Verification items for the finished model (mm, model axes). A direction names the side the tool comes from. Give positions to 0.01 mm unless a question says otherwise; leave off trailing zeros. Loops run counter-clockwise (first coordinate to the right, second up) from the corner with the lowest first, then second, coordinate; pieces in that order, holes last. Notation, with made-up numbers: (55.5, 28) - (81.5, 28) arc R10 cw to (81.5, 37) - close; hole circle Ø2 at (25, 22). An arc over 180 degrees is marked (long way). One line per item, written item: value. Start each with the question number.
1. Sectioned sample at A-A (x = 0.5). Record the cut outline in (y, z), plus the area to 3 significant figures.
2. Gauge pin test, flat ends, axial feed: pin 1 (2 mm diameter, centred on x = 17.5, y = 17.5, fed in from -Z); pin 2 (8.5 mm diameter, centred on x = -3, y = -1.5, fed in from -Z); pin 3 (1.4 mm diameter, centred on x = 17, y = 18, fed in from -Z); pin 4 (2.5 mm diameter, centred on y = -19, z = -3, fed in from -X). Record the tip position at first contact, or that the pin passes through.
3. Sectioned sample at C-C (y = -4). Record the cut outline in (x, z), plus the area to 3 significant figures.
4. Mould release check, pull along Y, two halves, no side actions. Record for faces 1 (the flat face through (15, 14, 0)), 2 (the cylindrical face through (16.002, 15.963, 4.493)), 3 (the flat face through (15, 0, -3.85)), 4 (the flat face through (-20, 0, 0)): pulls with the +Y half, pulls with the -Y half, needs draft (parallel to the pull), parting line crosses it, or undercut.
5. Scan lines: L1, parallel to Y at x = -17.5, z = 2.9; L2, parallel to Y at x = 17.5, z = 2.95; L3, parallel to Y at x = 0.5, z = -4.4. Record each from-to range of solid material in increasing order. Write a range as [from, to].
6. Sectioned sample at B-B (z = -2.5). Record the cut outline in (x, y), plus the area to 3 significant figures.
7. Sectioned sample at D-D (y = -8.5). Record the cut outline in (x, z).
8. Access from +Z, -Z, +X, -X, +Y, -Y to the whole of each face (thin tool, end or side, straight path). Record for faces 5 (the cylindrical face through (15.963, -16.002, 4.493)), 6 (the cylindrical face through (-15.963, 16.002, -1.796)), 7 (the flat face through (-18, 19, 4)), 8 (the flat face through (-19, -18, 4)).
from build123d import *

# Parameters (mm, degrees)
SKETCH_1_W          = 40
SKETCH_1_H          = 40
EXTRUDE_1_DEPTH     = 5
SKETCH_2_W          = 7.7
SKETCH_2_H          = 28
CUT_EXTRUDE_1_DEPTH = 10
CUT_EXTRUDE_2_DEPTH = 6.5
FILLET_1_R          = 2
CUT_EXTRUDE_START   = -1
CUT_EXTRUDE_3_DEPTH = 1
CUT_EXTRUDE_4_REACH = 31.682
SKETCH_5_R          = 1.189
SKETCH_6_R          = 14
CUT_EXTRUDE_5_DEPTH = 1


with BuildPart() as part:
    # 草图1 → 凸台-拉伸1 (new, symmetric)
    with BuildSketch(Plane.XY):
        Rectangle(SKETCH_1_W, SKETCH_1_H)
    extrude(amount=EXTRUDE_1_DEPTH, both=True)

    # 草图2 → 切除-拉伸1 (cut)
    with BuildSketch(Plane(origin=(20, 0, 0), x_dir=(0, 0, -1), z_dir=(1, 0, 0))):
        Rectangle(SKETCH_2_W, SKETCH_2_H)
    extrude(amount=-CUT_EXTRUDE_1_DEPTH, mode=Mode.SUBTRACT)

    # 草图3 → 切除-拉伸2 (cut)
    with BuildSketch(Plane(origin=(0, 0, -5), x_dir=(-1, 0, 0), z_dir=(0, 0, -1))):
        with BuildLine():
            Line((20, 20), (15.25, 20))
            Line((15.25, 20), (15.25, 17.75))
            ThreePointArc((15.25, 17.75), (15.982233047, 15.982233047), (17.75, 15.25))
            Line((17.75, 15.25), (20, 15.25))
            Line((20, 15.25), (20, 20))
        make_face()
        with BuildLine():
            Line((20, -20), (20, -15.25))
            Line((20, -15.25), (17.75, -15.25))
            ThreePointArc((17.75, -15.25), (15.982233047, -15.982233047), (15.25, -17.75))
            Line((15.25, -17.75), (15.25, -20))
            Line((15.25, -20), (20, -20))
        make_face()
        with BuildLine():
            Line((-17.75, -15.25), (-20, -15.25))
            Line((-20, -15.25), (-20, -20))
            Line((-20, -20), (-15.25, -20))
            Line((-15.25, -20), (-15.25, -17.75))
            ThreePointArc((-15.25, -17.75), (-15.982233047, -15.982233047), (-17.75, -15.25))
        make_face()
        with BuildLine():
            Line((-15.25, 17.75), (-15.25, 20))
            Line((-15.25, 20), (-20, 20))
            Line((-20, 20), (-20, 15.25))
            Line((-20, 15.25), (-17.75, 15.25))
            ThreePointArc((-17.75, 15.25), (-15.982233047, 15.982233047), (-15.25, 17.75))
        make_face()
    extrude(amount=-CUT_EXTRUDE_2_DEPTH, mode=Mode.SUBTRACT)

    # 圆角1
    fillet_1_edges = [part.edges().sort_by_distance(p)[0] for p in [
        (20, -20, 3.25),
        (-20, -20, 3.25),
        (-20, 20, 3.25),
        (20, 20, 3.25),
    ]]
    fillet(fillet_1_edges, radius=FILLET_1_R)

    # 草图4 → 切除-拉伸3 (cut)
    with BuildSketch(Plane.XY.offset(5).offset(CUT_EXTRUDE_START)):
        with BuildLine():
            Line((20, -15.25), (20, -18))
            ThreePointArc((20, -18), (19.414213562, -19.414213562), (18, -20))
            Line((18, -20), (15.25, -20))
            Line((15.25, -20), (15.25, -17.75))
            ThreePointArc((15.25, -17.75), (15.982233047, -15.982233047), (17.75, -15.25))
            Line((17.75, -15.25), (20, -15.25))
        make_face()
        with BuildLine():
            Line((-15.25, -20), (-18, -20))
            ThreePointArc((-18, -20), (-19.414213562, -19.414213562), (-20, -18))
            Line((-20, -18), (-20, -15.25))
            Line((-20, -15.25), (-17.75, -15.25))
            ThreePointArc((-17.75, -15.25), (-15.982233047, -15.982233047), (-15.25, -17.75))
            Line((-15.25, -17.75), (-15.25, -20))
        make_face()
        with BuildLine():
            Line((15.25, 20), (18, 20))
            ThreePointArc((18, 20), (19.414213562, 19.414213562), (20, 18))
            Line((20, 18), (20, 15.25))
            Line((20, 15.25), (17.75, 15.25))
            ThreePointArc((17.75, 15.25), (15.982233047, 15.982233047), (15.25, 17.75))
            Line((15.25, 17.75), (15.25, 20))
        make_face()
        with BuildLine():
            Line((-20, 15.25), (-20, 18))
            ThreePointArc((-20, 18), (-19.414213562, 19.414213562), (-18, 20))
            Line((-18, 20), (-15.25, 20))
            Line((-15.25, 20), (-15.25, 17.75))
            ThreePointArc((-15.25, 17.75), (-15.982233047, 15.982233047), (-17.75, 15.25))
            Line((-17.75, 15.25), (-20, 15.25))
        make_face()
    extrude(amount=CUT_EXTRUDE_3_DEPTH, mode=Mode.SUBTRACT)

    # 草图5 → 切除-拉伸4 (cut, up to next)
    with BuildSketch(Plane.XY.offset(4), mode=Mode.PRIVATE) as cut_extrude_4_sk1:
        with Locations((-17.5, 17.5)):
            Circle(SKETCH_5_R)
    cut_extrude_4_tool1 = extrude(cut_extrude_4_sk1.sketch, amount=-CUT_EXTRUDE_4_REACH, mode=Mode.PRIVATE) & part.part
    # 草图5 → 切除-拉伸4 (cut, up to next)
    with BuildSketch(Plane.XY.offset(4), mode=Mode.PRIVATE) as cut_extrude_4_sk2:
        with Locations(Location((-17.5, -17.5, 0), (0, 0, 180))):
            Circle(SKETCH_5_R)
    cut_extrude_4_tool2 = extrude(cut_extrude_4_sk2.sketch, amount=-CUT_EXTRUDE_4_REACH, mode=Mode.PRIVATE) & part.part
    # 草图5 → 切除-拉伸4 (cut, up to next)
    with BuildSketch(Plane.XY.offset(4), mode=Mode.PRIVATE) as cut_extrude_4_sk3:
        with Locations((17.5, -17.5)):
            Circle(SKETCH_5_R)
    cut_extrude_4_tool3 = extrude(cut_extrude_4_sk3.sketch, amount=-CUT_EXTRUDE_4_REACH, mode=Mode.PRIVATE) & part.part
    # 草图5 → 切除-拉伸4 (cut, up to next)
    with BuildSketch(Plane.XY.offset(4), mode=Mode.PRIVATE) as cut_extrude_4_sk4:
        with Locations(Location((17.5, 17.5, 0), (0, 0, 180))):
            Circle(SKETCH_5_R)
    cut_extrude_4_tool4 = extrude(cut_extrude_4_sk4.sketch, amount=-CUT_EXTRUDE_4_REACH, mode=Mode.PRIVATE) & part.part
    add(cut_extrude_4_tool1.solids().sort_by_distance((-17.5, 17.5, 4))[0], mode=Mode.SUBTRACT)
    add(cut_extrude_4_tool2.solids().sort_by_distance((-17.5, -17.5, 4))[0], mode=Mode.SUBTRACT)
    add(cut_extrude_4_tool3.solids().sort_by_distance((17.5, -17.5, 4))[0], mode=Mode.SUBTRACT)
    add(cut_extrude_4_tool4.solids().sort_by_distance((17.5, 17.5, 4))[0], mode=Mode.SUBTRACT)

    # 草图6 → 切除-拉伸5 (cut)
    with BuildSketch(Plane(origin=(0, 0, -5), x_dir=(-1, 0, 0), z_dir=(0, 0, -1))):
        with Locations((-0.5, -4)):
            Circle(SKETCH_6_R)
    extrude(amount=-CUT_EXTRUDE_5_DEPTH, mode=Mode.SUBTRACT)


solid = part.part
Results are:
1. outline: (-20, -5) - (-18, -5) - (-18, -4) - (10, -4) - (10, -5) - (20, -5) - (20, 5) - (-20, 5) - close
1. area: 372 mm^2
2. pin 1: passes through
2. pin 2: stops at z = -4
2. pin 3: stops at z = 1.5
2. pin 4: stops at x = -15.25
3. outline: (-20, -5) - (-13.5, -5) - (-13.5, -4) - (14.5, -4) - (14.5, -5) - (20, -5) - (20, -3.85) - (10, -3.85) - (10, 3.85) - (20, 3.85) - (20, 5) - (-20, 5) - close
3. area: 295 mm^2
4. face 1: undercut
4. face 2: pulls with the +Y half
4. face 3: undercut
4. face 4: needs draft
5. L1: y = [-20, -18.69], [-16.31, 16.31], [18.69, 20]
5. L2: y = [-20, -18.69], [-16.31, -14], [14, 16.31], [18.69, 20]
5. L3: y = [-20, -18], [10, 20]
6. outline: (-20, -15.25) - (-17.75, -15.25) arc R2.5 cw to (-15.25, -17.75) - (-15.25, -20) - (15.25, -20) - (15.25, -17.75) arc R2.5 cw to (17.75, -15.25) - (20, -15.25) - (20, -14) - (10, -14) - (10, 14) - (20, 14) - (20, 15.25) - (17.75, 15.25) arc R2.5 cw to (15.25, 17.75) - (15.25, 20) - (-15.25, 20) - (-15.25, 17.75) arc R2.5 cw to (-17.75, 15.25) - (-20, 15.25) - close
6. area: 1,240 mm^2
7. outline: (-20, -5) - (-12.76, -5) - (-12.76, -4) - (13.76, -4) - (13.76, -5) - (20, -5) - (20, -3.85) - (10, -3.85) - (10, 3.85) - (20, 3.85) - (20, 5) - (-20, 5) - close
8. face 5: +Z, +X, -Y
8. face 6: -Z, -X, +Y
8. face 7: +Z, -X, +Y
8. face 8: +Z, -X, -Y
